The listing builds one solid part. Answer for the finished solid, in the listing's coordinates (mm). Round coordinates to 2 decimals unless told otherwise and drop trailing zeros. Write each loop counter-clockwise with the first axis right and the second up, starting at its lowest first coordinate (ties: lowest second). Pieces come first, ordered by that corner, then holes. Notation, with made-up numbers: M -36,75.5 L -4,75.5 A20 cw -4,102.5 Z; hole C 82,23.25 d9. An arc over 180 degrees is marked long. One line per item, written item: value. Start each with the question number.
(1) Consider probe 1 along Y at (x, z) = (1.15, -2); probe 2 along Y at (x, z) = (-1.1, -2.5); probe 3 along Z at (x, y) = (-0.6, 19). Determine where each line is inside the solid, lowest interval first.
(2) Section A-A (x = -1.1) is taken. Determine the outline of the cut face in (y, z) (3 decimals), plus the area to 3 significant figures.
(3) Section B-B (y = 44) is taken. Determine the outline of the cut face in (x, z), plus the area to 3 significant figures.
(4) Section C-C (z = 36) is taken. Determine the outline of the cut face in (x, y), plus the area to 3 significant figures.
(5) Given P1, Ø1.5, axis at x = -1, z = 5, coming from the +Y side; P2, Ø1.5, axis at x = -0.5, y = 11.5, coming from the +Z side, each flat-ended and moving along its own axis, determine where each tip first touches the part or whether it passes through.
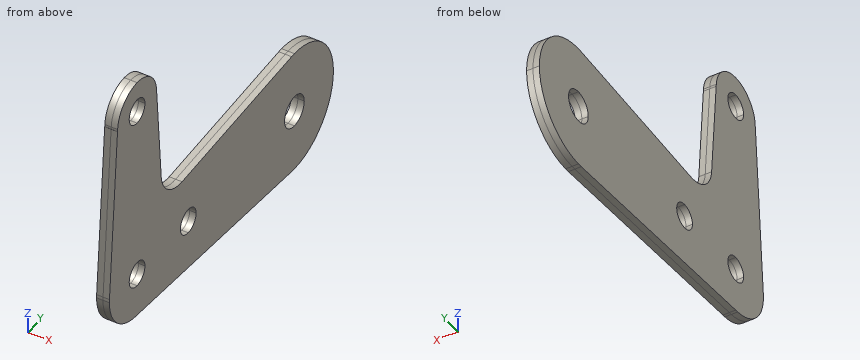
```python
from build123d import *

# Parameters (mm, degrees)
F1_DEPTH = 1.5875


with BuildPart() as f1:
    # F0 (on Right) → F1 (new body, symmetric)
    with BuildSketch(Plane.YZ):
        with BuildLine():
            Line((0, 41.275), (0, 3.175))
            ThreePointArc((0, 3.175), (2.2450640303, 2.2450640303), (3.175, 0))
            Line((3.175, 0), (17.4752, 0))
            ThreePointArc((17.4752, 0), (18.4051359697, 2.2450640303), (20.6502, 3.175))
            ThreePointArc((20.6502, 3.175), (22.8952640303, 2.2450640303), (23.8252, 0))
            Line((23.8252, 0), (59.5249, 0))
            ThreePointArc((59.5249, 0), (60.6891798341, 2.8108201659), (63.5, 3.9751))
            Line((63.5, 3.9751), (63.5, 15.748))
            ThreePointArc((63.5, 15.748), (62.9327037949, 15.7377787192), (62.366144, 15.7071281452))
            Line((62.366144, 15.7071281452), (18.1523895677, 12.515454258))
            ThreePointArc((18.1523895677, 12.515454258), (12.4398582326, 14.4089308884), (9.7332174357, 19.7840926163))
            Line((9.7332174357, 19.7840926163), (7.895816146, 44.45))
            Line((7.895816146, 44.45), (7.874, 44.45))
            Line((7.874, 44.45), (3.175, 44.45))
            ThreePointArc((3.175, 44.45), (2.2450640303, 42.2049359697), (0, 41.275))
        make_face()
        with BuildLine():
            Line((67.4751, 0), (79.248, 0))
            ThreePointArc((79.248, 0), (74.6355175901, 11.1355175901), (63.5, 15.748))
            Line((63.5, 15.748), (63.5, 3.9751))
            ThreePointArc((63.5, 3.9751), (66.3108201659, 2.8108201659), (67.4751, 0))
        make_face()
        with BuildLine():
            Line((63.5, -3.9751), (63.5, -15.748))
            ThreePointArc((63.5, -15.748), (74.6355175901, -11.1355175901), (79.248, 0))
            Line((79.248, 0), (67.4751, 0))
            ThreePointArc((67.4751, 0), (66.3108201659, -2.8108201659), (63.5, -3.9751))
        make_face()
        with BuildLine():
            ThreePointArc((3.175, 0), (2.2450640303, -2.2450640303), (0, -3.175))
            Line((0, -3.175), (0, -11.2050813091))
            Line((0, -11.2050813091), (62.366144, -15.7071281452))
            ThreePointArc((62.366144, -15.7071281452), (62.9327037949, -15.7377787192), (63.5, -15.748))
            Line((63.5, -15.748), (63.5, -3.9751))
            ThreePointArc((63.5, -3.9751), (60.6891798341, -2.8108201659), (59.5249, 0))
            Line((59.5249, 0), (23.8252, 0))
            ThreePointArc((23.8252, 0), (22.8952640303, -2.2450640303), (20.6502, -3.175))
            ThreePointArc((20.6502, -3.175), (18.4051359697, -2.2450640303), (17.4752, 0))
            Line((17.4752, 0), (3.175, 0))
        make_face()
        with BuildLine():
            ThreePointArc((-11.1451207035, 0.8302171429), (-11.1682775078, 0.4153956052), (-11.176, 0))
            Line((-11.176, 0), (-3.175, 0))
            ThreePointArc((-3.175, 0), (-2.2450640303, 2.2450640303), (0, 3.175))
            Line((0, 3.175), (0, 41.275))
            ThreePointArc((0, 41.275), (-2.2450640303, 42.2049359697), (-3.175, 44.45))
            Line((-3.175, 44.45), (-7.874, 44.45))
            Line((-7.874, 44.45), (-7.895816146, 44.45))
            Line((-7.895816146, 44.45), (-11.1451207035, 0.8302171429))
        make_face()
        with BuildLine():
            Line((-3.175, 0), (-11.176, 0))
            ThreePointArc((-11.176, 0), (-8.1821754525, -7.612816881), (-0.804672, -11.1469941676))
            Line((-0.804672, -11.1469941676), (0, -11.2050813091))
            Line((0, -11.2050813091), (0, -3.175))
            ThreePointArc((0, -3.175), (-2.2450640303, -2.2450640303), (-3.175, 0))
        make_face()
        with BuildLine():
            ThreePointArc((0, 47.625), (2.2450640303, 46.6950640303), (3.175, 44.45))
            Line((3.175, 44.45), (7.874, 44.45))
            ThreePointArc((7.874, 44.45), (7.8685591532, 44.7426650855), (7.852244132, 45.0349257143))
            ThreePointArc((7.852244132, 45.0349257143), (5.3569660689, 50.220857002), (0, 52.324))
            Line((0, 52.324), (0, 47.625))
        make_face()
        with BuildLine():
            ThreePointArc((-7.852244132, 45.0349257143), (-7.8685591532, 44.7426650855), (-7.874, 44.45))
            Line((-7.874, 44.45), (-3.175, 44.45))
            ThreePointArc((-3.175, 44.45), (-2.2450640303, 46.6950640303), (0, 47.625))
            Line((0, 47.625), (0, 52.324))
            ThreePointArc((0, 52.324), (-5.3569660689, 50.220857002), (-7.852244132, 45.0349257143))
        make_face()
    extrude(amount=F1_DEPTH, both=True)


solid = f1.part
```
Recorded:
1. probe 1: y = -11 to -2.47, 2.47 to 18.18, 23.12 to 60.06, 66.94 to 79.12
1. probe 2: y = -10.89 to -1.96, 1.96 to 18.69, 22.61 to 60.41, 66.59 to 79.05
1. probe 3: z = -12.58 to -2.71, 2.71 to 12.58
2. outline: M -11.145,0.83 A11.176 ccw -0.805,-11.147 L 62.366,-15.707 A15.748 ccw long 62.366,15.707 L 18.152,12.515 A7.874 cw 9.733,19.784 L 7.896,44.45 L 7.874,44.45 A7.874 ccw -7.874,44.45 L -7.896,44.45 Z; hole C 0,0 d6.35; hole C 0,44.45 d6.35; hole C 20.65,0 d6.35; hole C 63.5,0 d7.95
2. area: 2,890 mm2
3. outline: M -1.59,-14.38 L 1.59,-14.38 L 1.59,14.38 L -1.59,14.38 Z
3. area: 91.3 mm2
4. outline: M -1.59,-8.53 L 1.59,-8.53 L 1.59,8.53 L -1.59,8.53 Z
4. area: 54.1 mm2
5. P1: stops at y = 78.66
5. P2: stops at z = 16.46
